Geometry: see drawing. Coordinates: mm, zero at the bounding-box minimum. A direction names the side the tool comes from. Coordinates: 2 decimals unless noted, no trailing zeros. Write each loop counter-clockwise with the first axis right and the second up, starting at its lowest first coordinate (ties: lowest second). Pieces come first, ordered by that corner, then holes. Notation, with made-up numbers: (64, -31) - (81, -31) arc R17 cw to (81, 0) - close; hole circle Ø1 at (22, -30.75). An arc over 180 degrees is marked (long way). Use a Markdown table: item, result. Add a question column.
Q1. Section query D-D (y = 7). Return the cut outline in (x, z), then the cut area to 3 significant figures.
Q2. Material intervals for probe 1 along Y at (x, z) = (1, 4.25); probe 2 along X at (y, z) = (46.5, 6.25); probe 3 along X at (y, z) = (13.5, 9.25), sorted ascending. Write a range as from..to.
Q3. Section query A-A (x = 6). Return the cut outline in (y, z), then the cut area to 3 significant figures.
Q4. Set-up query: the marked faces 1, 2 and 3. Return all of +Z, -Z, +X, -X, +Y, -Y with unobstructed straight access to the full face (end or side cutting, diameter ignored); none if empty.
Q5. Section query C-C (y = 16.5). Return the cut outline in (x, z), then the cut area to 3 significant figures.
Q6. Pin query (flat end, axial travel): P1, Ø1.5, axis at x = 4.5, z = 2.5, coming from the -Y side; P2, Ø1, axis at x = 7.5, z = 3.5, coming from the +Y side; P3, Ø1, axis at x = 1.5, z = 4, coming from the +Y side. Return the tip coordinate at first contact, or that it passes through.
Q7. Section query B-B (z = 6). Return the cut outline in (x, y).
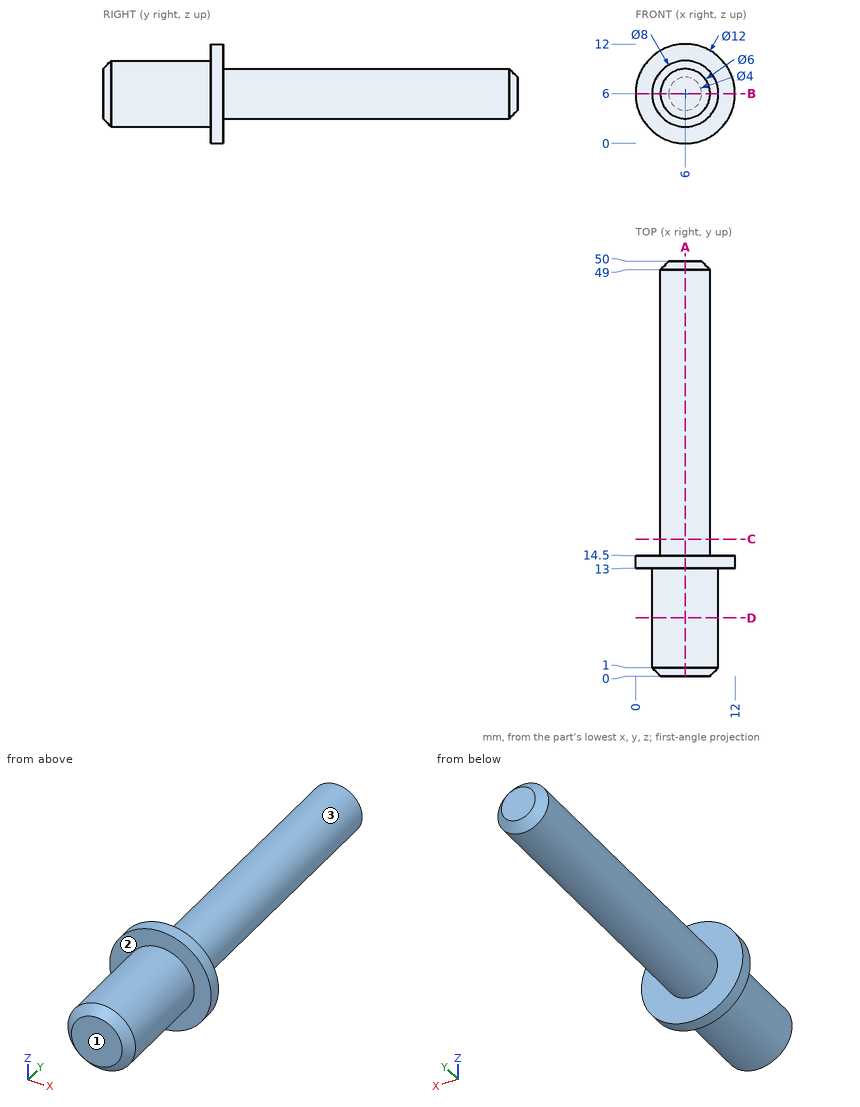
Values follow:
| question | item | result |
|---|---|---|
| 1 | outline | circle Ø8 at (6, 6) |
| 1 | area | 50.3 mm2 |
| 2 | probe 1 | 13..14.5 |
| 2 | probe 2 | 3.01..8.99 |
| 2 | probe 3 | 0.96..11.04 |
| 3 | outline | (0, 3) - (1, 2) - (13, 2) - (13, 0) - (14.5, 0) - (14.5, 3) - (49, 3) - (50, 4) - (50, 8) - (49, 9) - (14.5, 9) - (14.5, 12) - (13, 12) - (13, 10) - (1, 10) - (0, 9) - close |
| 3 | area | 333 mm2 |
| 4 | face 1 | +Z, -Z, +X, -X, -Y |
| 4 | face 2 | -Y |
| 4 | face 3 | +Y |
| 5 | outline | circle Ø6 at (6, 6) |
| 5 | area | 28.3 mm2 |
| 6 | P1 | y = 0.06 |
| 6 | P2 | y = 49.58 |
| 6 | P3 | y = 14.5 |
| 7 | outline | (0, 13) - (2, 13) - (2, 1) - (3, 0) - (9, 0) - (10, 1) - (10, 13) - (12, 13) - (12, 14.5) - (9, 14.5) - (9, 49) - (8, 50) - (4, 50) - (3, 49) - (3, 14.5) - (0, 14.5) - close |
